Print and shaded views of the part. All mm, measured from the part's lowest x, y and z. A direction names the side the tool comes from. Round coordinates to 2 decimals unless told otherwise and drop trailing zeros. Write each loop counter-clockwise with the first axis right and the second up, starting at its lowest first coordinate (ties: lowest second). Pieces come first, ordered by that corner, then holes. Notation, with made-up numbers: (13, 71.25) - (51, 71.25) arc R6 cw to (51, 78.25) - close; hole circle Ø8 at (-12.5, 80). An arc over 180 degrees is marked (long way). One line per item, written item: value.
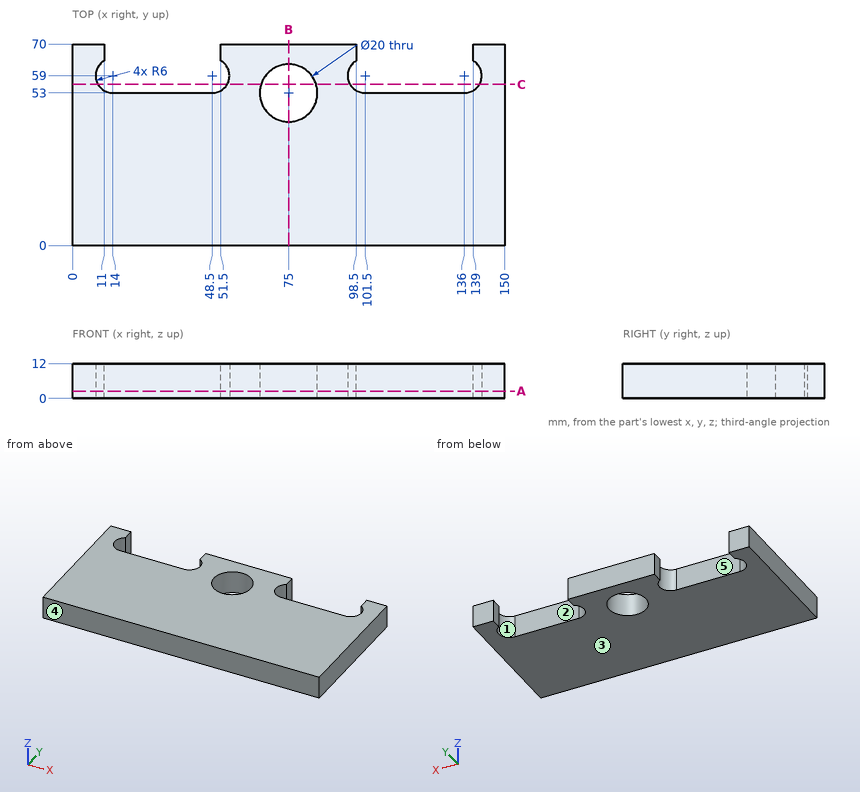
1. Mould opens along X. For the marked faces 4 and 5 say: released by +X, released by -X, zero draft, split by the parting line, or undercut.
Report:
face 4: zero draft
face 5: undercut
2. Wall check: probe 1 along Y at (x, z) = (75, 2.75); probe 2 along X at (y, z) = (55, 5); probe 3 along X at (y, z) = (64, 10.5). Give the ranges that are in metal, low to high. Write a range as [from, to].
Report:
probe 1: [0, 43], [63, 70]
probe 2: [0, 9.53], [52.97, 65.2], [84.8, 97.03], [140.47, 150]
probe 3: [0, 10.68], [51.82, 98.18], [139.32, 150]
3. Band-saw the part on A-A on z = 2.5. Write the cut outline in (x, y), plus the area to 3 significant figures.
Report:
outline: (0, 0) - (150, 0) - (150, 70) - (139, 70) - (139, 64.2) arc R6 cw to (136, 53) - (101.5, 53) arc R6 cw to (98.5, 64.2) - (98.5, 70) - (51.5, 70) - (51.5, 64.2) arc R6 cw to (48.5, 53) - (14, 53) arc R6 cw to (11, 64.2) - (11, 70) - (0, 70) - close; hole circle Ø20 at (75, 53)
area: 8,720 mm²
4. Band-saw the part on B-B on x = 75. Write the cut outline in (y, z).
Report:
outline: (0, 0) - (43, 0) - (43, 12) - (0, 12) - close; (63, 0) - (70, 0) - (70, 12) - (63, 12) - close
5. Tool access for the marked faces 1, 2 and 3: list every direction of +Z, -Z, +X, -X, +Y, -Y with a clear straight run to the whole face (end or side of a thin tool).
Report:
face 1: +Z, -Z
face 2: +Z, -Z, +Y
face 3: -Z, +X, -X, +Y, -Y
6. Band-saw the part on C-C on y = 56. Write the cut outline in (x, z), plus the area to 3 significant figures.
Report:
outline: (0, 0) - (8.8, 0) - (8.8, 12) - (0, 12) - close; (53.7, 0) - (65.46, 0) - (65.46, 12) - (53.7, 12) - close; (84.54, 0) - (96.3, 0) - (96.3, 12) - (84.54, 12) - close; (141.2, 0) - (150, 0) - (150, 12) - (141.2, 12) - close
area: 494 mm²
7. Drop a flat-ended pin along its axis: pin 1 (1.5 mm diameter, centred on x = 48.5, z = 9, fed in from +Y). Give the stop position or say it passes through.
Report:
pin 1: y = 53.05
